Verification items for the finished model (mm, model axes). Give positions to 0.01 mm unless a question says otherwise; leave off trailing zeros. Order: outer loops, then holes, each group sorted by start corner. A loop starts at its lowest first (then second) coordinate and runs counter-clockwise, first axis right, second up. Notation, with made-up numbers: (-15.75, 83.25) -> (22.25, 83.25) arc R7 cw to (22.25, 91.25) -> close; hole circle Ø4 at (77.25, 80.25). An arc over 180 degrees is marked (long way). Return JSON: item names as keys, results as strings. Group by question number.
(1) Cross-section at B-B on x = 50.8. Enter the section's corners in (y, z) (3 decimals), then the cut area to 3 significant figures.
(2) Cross-section at C-C on z = 50.8. Enter the section's corners in (x, y) (3 decimals).
(3) Cross-section at A-A on y = -7.75. Enter the section's corners in (x, z).
(4) Depth check by flat-ended pin: pin 1 Ø4 at (x, z) = (-50.8, -50.8) entering from +Y; pin 2 Ø11.5 at (x, z) = (50.8, -50.8) entering from -Y (3 decimals). Enter the tip coordinate at first touch or a pass-through.
(5) Thickness scan on line 1 along Z through (x, y) = (50.8, -5.25); line 2 along Z through (x, y) = (50.8, 0.5) (3 decimals); line 3 along X through (y, z) = (-4.25, 53). Record the ranges inside material, lowest first.
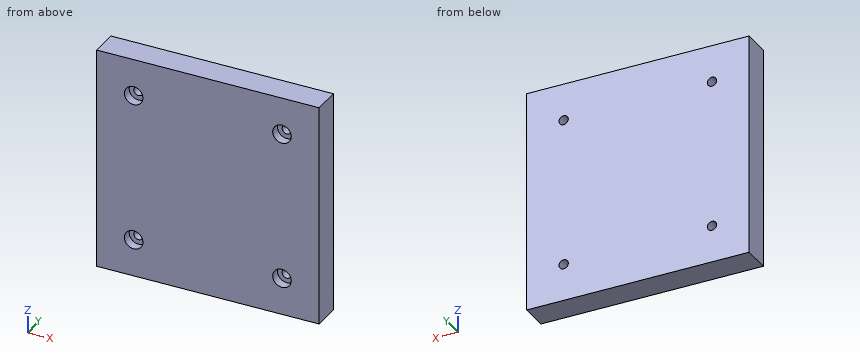
from build123d import *

# Parameters (mm, degrees)
F0_W           = 152.4
F0_H           = 152.4
F1_DEPTH       = 9.525
F3_D           = 6.35
F3_CBORE_D     = 12.7
F3_CBORE_DEPTH = 6.35


with BuildPart() as f1:
    # F0 (on Front) → F1 (new body, symmetric)
    with BuildSketch(Plane.XZ):
        Rectangle(F0_W, F0_H)
    extrude(amount=F1_DEPTH, both=True)

    # F3 (through all)
    with Locations(Plane.XZ.offset(9.525)):
        with Locations((-50.8, 50.8), (50.8, 50.8), (50.8, -50.8), (-50.8, -50.8)):
            CounterBoreHole(F3_D / 2, F3_CBORE_D / 2, F3_CBORE_DEPTH)


solid = f1.part
Verdict:
{
 "1": {"outline": "(-9.525, -76.2) -> (9.525, -76.2) -> (9.525, -53.975) -> (-3.175, -53.975) -> (-3.175, -57.15) -> (-9.525, -57.15) -> close; (-9.525, -44.45) -> (-3.175, -44.45) -> (-3.175, -47.625) -> (9.525, -47.625) -> (9.525, 47.625) -> (-3.175, 47.625) -> (-3.175, 44.45) -> (-9.525, 44.45) -> close; (-9.525, 57.15) -> (-3.175, 57.15) -> (-3.175, 53.975) -> (9.525, 53.975) -> (9.525, 76.2) -> (-9.525, 76.2) -> close", "area": "2,580 mm²"},
 "2": {"outline": "(-76.2, -9.525) -> (-57.15, -9.525) -> (-57.15, -3.175) -> (-53.975, -3.175) -> (-53.975, 9.525) -> (-76.2, 9.525) -> close; (-47.625, -3.175) -> (-44.45, -3.175) -> (-44.45, -9.525) -> (44.45, -9.525) -> (44.45, -3.175) -> (47.625, -3.175) -> (47.625, 9.525) -> (-47.625, 9.525) -> close; (53.975, -3.175) -> (57.15, -3.175) -> (57.15, -9.525) -> (76.2, -9.525) -> (76.2, 9.525) -> (53.975, 9.525) -> close"},
 "3": {"outline": "(-76.2, -76.2) -> (76.2, -76.2) -> (76.2, 76.2) -> (-76.2, 76.2) -> close; hole circle Ø12.7 at (-50.8, -50.8); hole circle Ø12.7 at (-50.8, 50.8); hole circle Ø12.7 at (50.8, -50.8); hole circle Ø12.7 at (50.8, 50.8)"},
 "4": {"pin 1": "through", "pin 2": "y = -3.175"},
 "5": {"line 1": "-76.2 to -57.15, -44.45 to 44.45, 57.15 to 76.2", "line 2": "-76.2 to -53.975, -47.625 to 47.625, 53.975 to 76.2", "line 3": "-76.2 to -56.76, -44.84 to 44.84, 56.76 to 76.2"}
}
